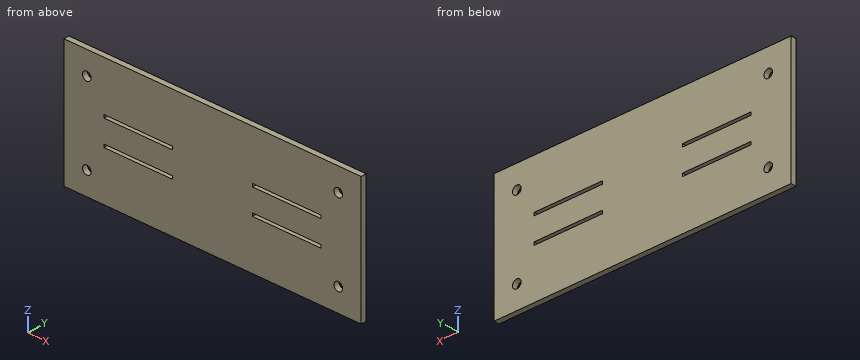
```python
from build123d import *

# Parameters (mm, degrees)
SKETCH1_W           = 165.1
SKETCH1_H           = 69.85
BOSS_EXTRUDE1_DEPTH = 3
CUT_EXTRUDE3_REACH  = 91.684
SKETCH8_R           = 2.38125
SKETCH10_W          = 38.1
SKETCH10_H          = 1.651
CUT_EXTRUDE4_DEPTH  = 26.67


with BuildPart() as part:
    # Sketch1 → Boss-Extrude1 (new body)
    with BuildSketch(Plane(origin=(0, 0, 0), x_dir=(1, 0, 0), z_dir=(0, 1, 0))):
        Rectangle(SKETCH1_W, SKETCH1_H)
    extrude(amount=BOSS_EXTRUDE1_DEPTH)

    # Sketch8 → Cut-Extrude3 (cut, up to next)
    with BuildSketch(Plane(origin=(0, 3, 0), x_dir=(1, 0, 0), z_dir=(0, 1, 0)), mode=Mode.PRIVATE) as cut_extrude3_sk1:
        with Locations(Location((-69.85, -22.225, 0), (0, 0, 270))):
            Circle(SKETCH8_R)
    cut_extrude3_tool1 = extrude(cut_extrude3_sk1.sketch, amount=-CUT_EXTRUDE3_REACH, mode=Mode.PRIVATE) & part.part
    # Sketch8 → Cut-Extrude3 (cut, up to next)
    with BuildSketch(Plane(origin=(0, 3, 0), x_dir=(1, 0, 0), z_dir=(0, 1, 0)), mode=Mode.PRIVATE) as cut_extrude3_sk2:
        with Locations(Location((-69.85, 22.225, 0), (0, 0, 270))):
            Circle(SKETCH8_R)
    cut_extrude3_tool2 = extrude(cut_extrude3_sk2.sketch, amount=-CUT_EXTRUDE3_REACH, mode=Mode.PRIVATE) & part.part
    # Sketch8 → Cut-Extrude3 (cut, up to next)
    with BuildSketch(Plane(origin=(0, 3, 0), x_dir=(1, 0, 0), z_dir=(0, 1, 0)), mode=Mode.PRIVATE) as cut_extrude3_sk3:
        with Locations(Location((69.85, 22.225, 0), (0, 0, 270))):
            Circle(SKETCH8_R)
    cut_extrude3_tool3 = extrude(cut_extrude3_sk3.sketch, amount=-CUT_EXTRUDE3_REACH, mode=Mode.PRIVATE) & part.part
    # Sketch8 → Cut-Extrude3 (cut, up to next)
    with BuildSketch(Plane(origin=(0, 3, 0), x_dir=(1, 0, 0), z_dir=(0, 1, 0)), mode=Mode.PRIVATE) as cut_extrude3_sk4:
        with Locations(Location((69.85, -22.225, 0), (0, 0, 270))):
            Circle(SKETCH8_R)
    cut_extrude3_tool4 = extrude(cut_extrude3_sk4.sketch, amount=-CUT_EXTRUDE3_REACH, mode=Mode.PRIVATE) & part.part
    add(cut_extrude3_tool1.solids().sort_by_distance((-69.85, 3, 22.225))[0], mode=Mode.SUBTRACT)
    add(cut_extrude3_tool2.solids().sort_by_distance((-69.85, 3, -22.225))[0], mode=Mode.SUBTRACT)
    add(cut_extrude3_tool3.solids().sort_by_distance((69.85, 3, -22.225))[0], mode=Mode.SUBTRACT)
    add(cut_extrude3_tool4.solids().sort_by_distance((69.85, 3, 22.225))[0], mode=Mode.SUBTRACT)

    # Sketch10 → Cut-Extrude4 (cut)
    with BuildSketch(Plane.XZ):
        with Locations((-41.275, -6.985)):
            Rectangle(SKETCH10_W, SKETCH10_H)
        with Locations((-41.275, 6.985)):
            Rectangle(SKETCH10_W, SKETCH10_H)
        with Locations((41.275, 6.985)):
            Rectangle(SKETCH10_W, SKETCH10_H)
        with Locations((41.275, -6.985)):
            Rectangle(SKETCH10_W, SKETCH10_H)
    extrude(amount=-CUT_EXTRUDE4_DEPTH, mode=Mode.SUBTRACT)


solid = part.part
```
Here's how the part is built. I have some questions about the finished solid (model axes, mm). Round coordinates to 2 decimals unless told otherwise and drop trailing zeros. Order: outer loops, then holes, each group sorted by start corner. A loop starts at its lowest first (then second) coordinate and runs counter-clockwise, first axis right, second up. Notation, with made-up numbers: M -9,54 L 46,54 A27 ccw 46,72 Z; hole C 33,66 d11. An arc over 180 degrees is marked long. Use CSV: the item, a comma, the result in double quotes.
1) I need wall thicknesses on line 1 along Z through (x, y) = (44, 1.5) (1 decimal); line 2 along X through (y, z) = (1.35, -22); line 3 along X through (y, z) = (2.3, -24). Which ranges of each line are inside material? Lowest first, please. Write a range as [from, to].
Taken from the geometry:
line 1,"[-34.9, -7.8], [-6.2, 6.2], [7.8, 34.9]"
line 2,"[-82.55, -72.22], [-67.48, 67.48], [72.22, 82.55]"
line 3,"[-82.55, -71.44], [-68.26, 68.26], [71.44, 82.55]"
2) I want a section at C-C (x = -69.85). List the corners of the cut face in (y, z) for me (3 decimals).
Taken from the geometry:
outline,"M 0,-34.925 L 3,-34.925 L 3,-24.606 L 0,-24.606 Z; M 0,-19.844 L 3,-19.844 L 3,19.844 L 0,19.844 Z; M 0,24.606 L 3,24.606 L 3,34.925 L 0,34.925 Z"
3) I want a section at B-B (y = 0.8). Count the separate pieces of the cut face and the enclosed holes in it, then the cut area to 3 significant figures.
Taken from the geometry:
separate pieces,"1"
enclosed holes,"8"
area,"11,200 mm^2"
4) I want a section at A-A (x = -44.5). List the corners of the cut face in (y, z) for me (1 decimal), then the cut area to 3 significant figures.
Taken from the geometry:
outline,"M 0,-34.9 L 3,-34.9 L 3,-7.8 L 0,-7.8 Z; M 0,-6.2 L 3,-6.2 L 3,6.2 L 0,6.2 Z; M 0,7.8 L 3,7.8 L 3,34.9 L 0,34.9 Z"
area,"200 mm^2"
